Part model, mm, in its own coordinate system. Face numbers are marked on the shaded views. A direction names the side the tool comes from. Round coordinates to 2 decimals unless told otherwise and drop trailing zeros. Loops run counter-clockwise (first coordinate to the right, second up) from the corner with the lowest first, then second, coordinate; pieces in that order, holes last.
Autodesk Inventor part; units mm, degrees
ref_plane "Work Plane2" through (0, 0, 1.5) normal (0, 0, 1) x (1, 0, 0)
ref_plane "Work Plane8" through (0, 0, 0) normal (0.9510565, 0.309017, 0) x (0, 0, 1)
ref_plane "Work Plane9" through (0, 0, 0) normal (1, 0, 0) x (0, 1, 0)
sketch "Sketch1" plane through (0, 0, 0) normal (0, 0, 1) x (1, 0, 0)
  circle A0 centre (0, 0) radius 12.2166
  dimension "d0" = 24.4331
extrude "Extrusion1" add sketch "Sketch1" along normal blind 3
ref_plane "Work Plane2" through (0, 0, 1.5) normal (0, 0, 1) x (1, 0, 0)
sketch "Sketch2" plane through (0, 0, 0) normal (0, 0, -1) x (-1, 0, 0)
  circle A0 centre (0, 0) radius 12.2166
  circle A1 centre (0, 0) radius 10
  dimension "d3" = 20
surface extrude "Средний диаметр" sketch "Sketch2" against normal through all shown no curves A1
ref_plane "Work Plane8" through (0, 0, 0) normal (0.9510565, 0.309017, 0) x (0, 0, 1)
ref_plane "Work Plane9" through (0, 0, 0) normal (1, 0, 0) x (0, 1, 0)
spur gear teeth "Цилиндрическое зубчатое зацепление" teeth 10 pitch diameter 20 tip diameter 24.4331 root diameter 15.4331 face width 3 start plane through (0, 0, 0) normal (0, 0, -1) x (-1, 0, 0)
equation "\"d0\" = da_da"
equation "\"d1\" = da_b"
equation "\"d3\" = da_d"
properties part number "Цилиндрическое зубчатое зацепление1" material "Steel"
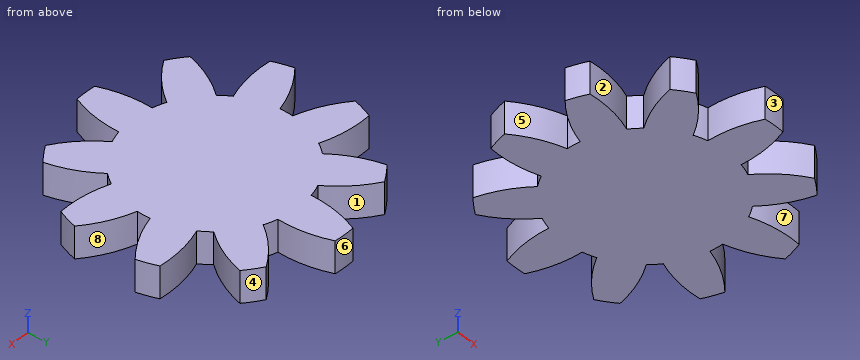
1) Slice it at C-C, the plane x = 4.75. Give the cut face in (y, z).
Values:
outline: (-9.2, 0) - (9.2, 0) - (9.2, 3) - (-9.2, 3) - close
2) Slice it at B-B, the plane x = 8.5. Give the cut face in (y, z), then the cut area to 3 significant figures.
Values:
outline: (-4.55, 0) - (-0.87, 0) - (-0.87, 3) - (-4.55, 3) - close; (0.87, 0) - (4.55, 0) - (4.55, 3) - (0.87, 3) - close
area: 22.1 mm2
3) Tool access for the marked faces 4, 5, 6, 7 and 8: list every direction of +Z, -Z, +X, -X, +Y, -Y with a clear straight run to the whole face (end or side of a thin tool).
Values:
face 4: +Z, -Z, +X, +Y
face 5: +Z, -Z, -X
face 6: +Z, -Z, +Y
face 7: +Z, -Z
face 8: +Z, -Z, +X
4) Slice it at D-D, the plane y = 1.25. Give the cut face in (x, z).
Values:
outline: (-9.42, 0) - (9.42, 0) - (9.42, 3) - (-9.42, 3) - close
5) Wall check: line 1 along X through (y, z) = (9.25, 0.75); line 2 along X through (y, z) = (-8.25, 2.5); line 3 along Y through (x, z) = (-0.25, 0.7). Give the ranges that are in metal, low to high.
Values:
line 1: x = -7.92 to -4.8, -1.73 to 1.73, 4.8 to 7.92
line 2: x = -7.63 to -3.81, -1.81 to 1.81, 3.81 to 7.63
line 3: y = -12.21 to 12.21
6) Mould opens along Y. For the marked faces 1, 2 and 3 say: released by +Y, released by -Y, zero draft, split by the parting line, or undercut.
Values:
face 1: released by +Y
face 2: undercut
face 3: released by -Y
7) Slice it at A-A, the plane y = 8.75. Give the cut face in (x, z).
Values:
outline: (-7.79, 0) - (-4.27, 0) - (-4.27, 3) - (-7.79, 3) - close; (-1.78, 0) - (1.78, 0) - (1.78, 3) - (-1.78, 3) - close; (4.27, 0) - (7.79, 0) - (7.79, 3) - (4.27, 3) - close
8) Drop flat-ended pins along their axis: pin 1 Ø1.5 at (y, z) = (9, 2.5) entering from -X; pin 2 Ø1 at (x, y) = (-6, 0.5) entering from -Z; pin 3 Ø1 at (x, z) = (-5.5, 0.5) entering from -Y. Give the stop position or say it passes through.
Values:
pin 1: stops at x = -7.93
pin 2: stops at z = 0
pin 3: stops at y = -10.17
